```python
from build123d import *

# Parameters (mm, degrees)
EXTRUDE_476_DEPTH          = 25
CUT_EXTRUDE_647_DEPTH      = 27.815775829
CUT_EXTRUDE_647_DEPTH_BACK = 27.815775829
SKETCH_8_R                 = 8.875
SKETCH_8_R_2               = 6.875
CUT_EXTRUDE_851_DEPTH      = 27.694346312
CUT_EXTRUDE_851_DEPTH_BACK = 27.694346312
SKETCH_9_R                 = 2.55


with BuildPart() as part:
    # 草图1 → Extrude 476 (new, symmetric)
    with BuildSketch(Plane(origin=(0, 0, 0), x_dir=(0, 0, -1), z_dir=(1, 0, 0))):
        Polygon((7.332348419, 0), (3.666174209, 6.35), (-3.666174209, 6.35), (-7.332348419, 0), (-3.666174209, -6.35), (3.666174209, -6.35), align=None)
    extrude(amount=EXTRUDE_476_DEPTH, both=True)

    # 草图8 → Cut-Extrude 647 (cut, two sides: drawn at the far end of the back side and taken through both)
    with BuildSketch(Plane(origin=(0, 0, 0), x_dir=(0, 0, -1), z_dir=(1, 0, 0)).offset(-CUT_EXTRUDE_647_DEPTH_BACK)):
        Circle(SKETCH_8_R)
        Circle(SKETCH_8_R_2, mode=Mode.SUBTRACT)
    extrude(amount=CUT_EXTRUDE_647_DEPTH + CUT_EXTRUDE_647_DEPTH_BACK, mode=Mode.SUBTRACT)

    # 草图9 → Cut-Extrude 851 (cut, two sides: drawn at the far end of the back side and taken through both)
    with BuildSketch(Plane(origin=(0, 0, 0), x_dir=(0, 0, -1), z_dir=(1, 0, 0)).offset(-CUT_EXTRUDE_851_DEPTH_BACK)):
        Circle(SKETCH_9_R)
    extrude(amount=CUT_EXTRUDE_851_DEPTH + CUT_EXTRUDE_851_DEPTH_BACK, mode=Mode.SUBTRACT)

    # 草图10 → Cut-Revolve 1145 (revolve, cut)
    with BuildSketch(Plane.XY, mode=Mode.PRIVATE) as cut_revolve_1145_sk:
        Polygon((-26, 7.35), (-23, 7.35), (-26, 4.35), align=None)
        Polygon((23, 7.35), (26, 4.35), (26, 7.35), align=None)
    revolve(cut_revolve_1145_sk.sketch.rotate(Axis((25, 0, 0), (-1, 0, 0)), 157.463629785), axis=Axis((25, 0, 0), (-1, 0, 0)), mode=Mode.SUBTRACT)


solid = part.part
```
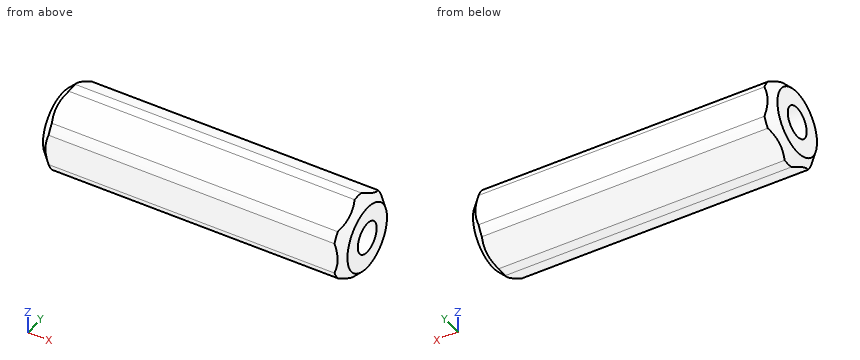
Work out the finished part from the listing and answer in its coordinate system (mm). Give positions to 0.01 mm unless a question says otherwise; leave off trailing zeros. Loops run counter-clockwise (first coordinate to the right, second up) from the corner with the lowest first, then second, coordinate; pieces in that order, holes last. Notation, with made-up numbers: (63.25, 17.25) -> (113.25, 17.25) arc R23 cw to (113.25, 35.25) -> close; hole circle Ø1 at (46, 72). An arc over 180 degrees is marked (long way). One line per question, with ' | ' between items. Start each with the question number.
1) Section C-C, the plane x = -1 is taken. Determine the outline of the cut face in (y, z) (3 decimals), then the cut area to 3 significant figures.
2) Straight lines are drawn through the part: L1, parallel to Z at x = 2.5, y = 0 (3 decimals); L2, parallel to Y at x = -0.5, z = 0; L3, parallel to Y at x = 16, z = 0.75. For each, find the intervals that lie inside material, in ascending order.
3) Section B-B, the plane z = 0 is taken. Determine the outline of the cut face in (x, y).
4) Section A-A, the plane y = 0 is taken. Determine the outline of the cut face in (x, z) (3 decimals), then the cut area to 3 significant figures.
Resolved:
1) outline: (-6.35, -2.635) arc R6.875 ccw to (-5.457, -4.182) -> (-0.893, -6.817) arc R6.875 ccw to (0.893, -6.817) -> (5.457, -4.182) arc R6.875 ccw to (6.35, -2.635) -> (6.35, 2.635) arc R6.875 ccw to (5.457, 4.182) -> (0.893, 6.817) arc R6.875 ccw to (-0.893, 6.817) -> (-5.457, 4.182) arc R6.875 ccw to (-6.35, 2.635) -> close; hole circle Ø5.1 at (0, 0) | area: 117 mm2
2) L1: -6.875 to -2.55, 2.55 to 6.875 | L2: -6.35 to -2.55, 2.55 to 6.35 | L3: -6.35 to -2.44, 2.44 to 6.35
3) outline: (-25, -5.35) -> (-24, -6.35) -> (24, -6.35) -> (25, -5.35) -> (25, -2.55) -> (-25, -2.55) -> close; (-25, 2.55) -> (25, 2.55) -> (25, 5.35) -> (24, 6.35) -> (-24, 6.35) -> (-25, 5.35) -> close
4) outline: (-25, -5.35) -> (-23.475, -6.875) -> (23.475, -6.875) -> (25, -5.35) -> (25, -2.55) -> (-25, -2.55) -> close; (-25, 2.55) -> (25, 2.55) -> (25, 5.35) -> (23.475, 6.875) -> (-23.475, 6.875) -> (-25, 5.35) -> close | area: 428 mm2
